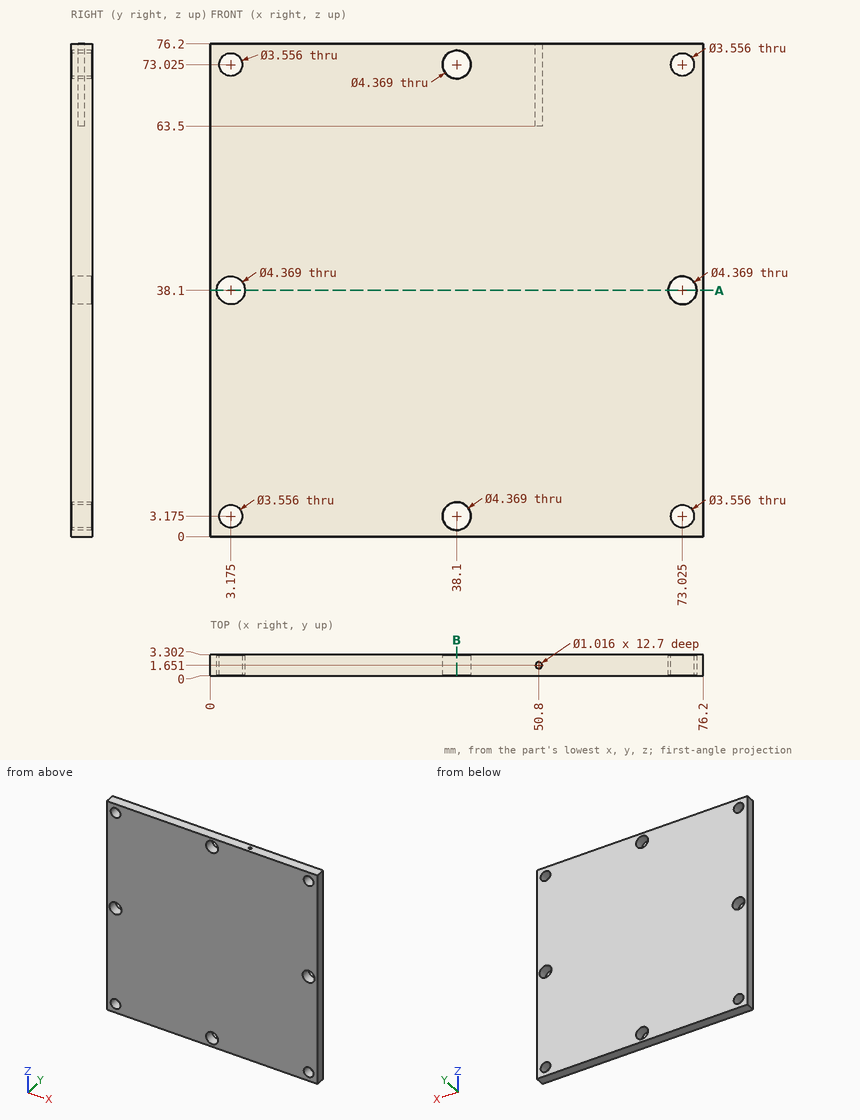
Print and shaded views of the part. All mm, measured from the part's lowest x, y and z. Give positions to 0.01 mm unless a question says otherwise; leave off trailing zeros. Write each loop counter-clockwise with the first axis right and the second up, starting at its lowest first coordinate (ties: lowest second). Pieces come first, ordered by that corner, then holes. Notation, with made-up numbers: (-2.5, 50.25) - (4.5, 50.25) arc R36 cw to (4.5, 85.25) - close; hole circle Ø8 at (-36, 82.5). An arc over 180 degrees is marked (long way). Put each result on its own line as item: value.
(1) Wall check: L1, parallel to Z at x = 73, y = 1.3; L2, parallel to Z at x = 40, y = 1.2; L3, parallel to X at y = 0.8, z = 37.5 (1 decimal). Give the ranges that are in metal, low to high.
Working result:
L1: 0 to 1.4, 4.95 to 35.92, 40.28 to 71.25, 74.8 to 76.2
L2: 0 to 2.1, 4.25 to 71.95, 74.1 to 76.2
L3: 0 to 1.1, 5.3 to 70.9, 75.1 to 76.2
(2) Saw through at A-A (z = 38.1). List the corners of the cut face in (x, y).
Working result:
outline: (0, 0) - (0.99, 0) - (0.99, 3.3) - (0, 3.3) - close; (5.36, 0) - (70.84, 0) - (70.84, 3.3) - (5.36, 3.3) - close; (75.21, 0) - (76.2, 0) - (76.2, 3.3) - (75.21, 3.3) - close
(3) Saw through at B-B (x = 38.1). List the corners of the cut face in (y, z).
Working result:
outline: (0, 0) - (3.3, 0) - (3.3, 0.99) - (0, 0.99) - close; (0, 5.36) - (3.3, 5.36) - (3.3, 70.84) - (0, 70.84) - close; (0, 75.21) - (3.3, 75.21) - (3.3, 76.2) - (0, 76.2) - close
